Study the drawing (mm; zero at the part's minimum x, y, z) and answer. A direction names the side the tool comes from. Round coordinates to 2 decimals unless told otherwise and drop trailing zeros. Order: outer loops, then holes, each group sorted by start corner. A loop starts at its lowest first (then second) coordinate and runs counter-clockwise, first axis right, second up. Notation, with made-up numbers: M -26.75,71.5 L -12.75,71.5 A8 cw -12.75,83.5 Z; hole C 65.25,49.25 d9. An arc over 180 degrees is marked long. Put each result on its own line as item: value. Start each with the question number.
1. The mould has two halves that part along Y. Classify the marked faces 1, 2 and 3: +Y half, -Y half, draft (parallel to the pull), parting line (faces both ways), or undercut.
2. The part is cut by section A-A (z = 17). Give the vertices of the cut face in (x, y), then the cut area to 3 significant figures.
3. The part is cut by section B-B (x = 5). Give the vertices of the cut face in (y, z), then the cut area to 3 significant figures.
4. Each of these flat-tipped pins is pushed along its axis until it touches: pin 1 Ø5 at (y, z) = (11.5, 15.5) entering from -X; pin 2 Ø3 at (y, z) = (6, 20) entering from +X; pin 3 Ø5 at (x, y) = (24, 8) entering from -Z; pin 4 Ø3 at (x, z) = (6.5, 17.5) entering from +Y. Where does it stop, or does it pass through?
5. The part is cut by section C-C (z = 10.25). Give the vertices of the cut face in (x, y).
6. Which of the six approach directions +Z, -Z, +X, -X, +Y, -Y give full straight-line access (tool end or side, diameter ignored) to the marked faces 4, 5 and 6?
7. Consider line 1 (X direction, y = 1, z = 17); line 2 (X direction, y = 10, z = 17.75); line 3 (X direction, y = 5, z = 11.25). Determine where each line is inside the solid, lowest interval first.
8. The part is cut by section D-D (y = 14). Give the vertices of the cut face in (x, z), then the cut area to 3 significant figures.
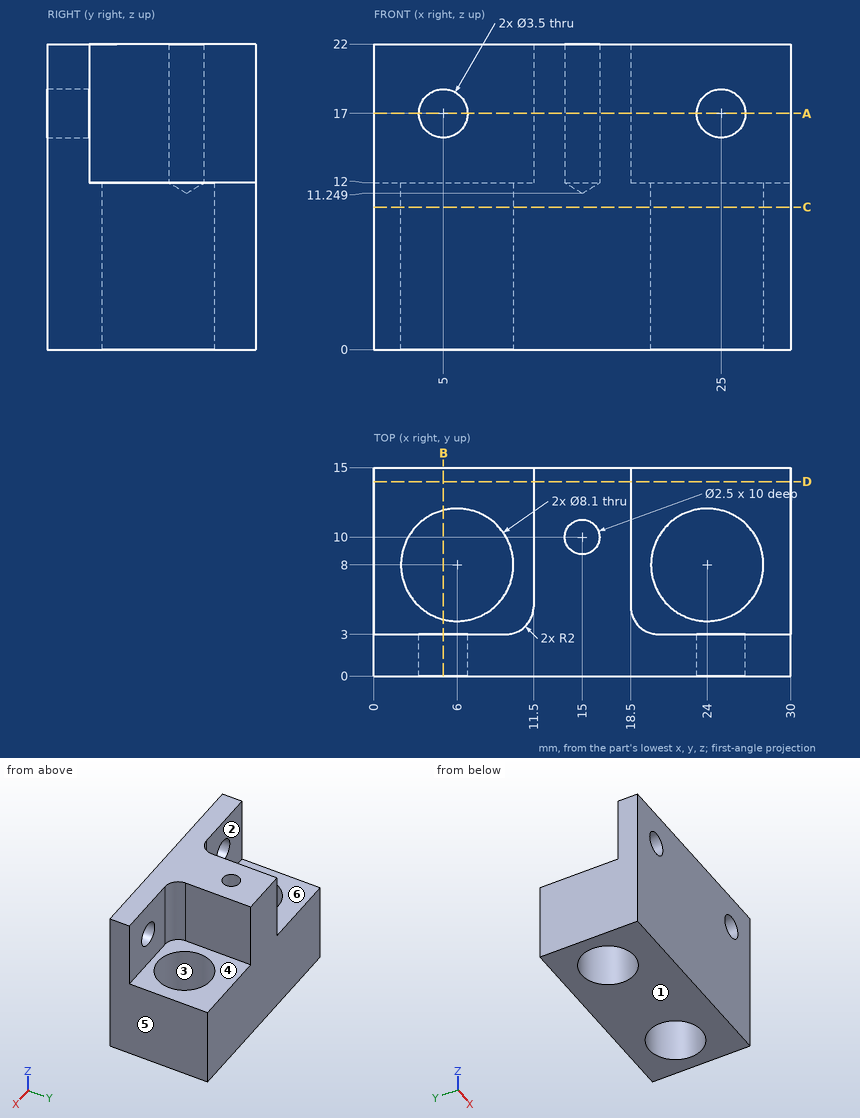
Resolved:
1. face 1: draft
1. face 2: +Y half
1. face 3: undercut
2. outline: M 0,0 L 3.25,0 L 3.25,3 L 0,3 Z; M 6.75,0 L 23.25,0 L 23.25,3 L 20.5,3 A2 cw 18.5,5 L 18.5,15 L 11.5,15 L 11.5,5 A2 cw 9.5,3 L 6.75,3 Z; M 26.75,0 L 30,0 L 30,3 L 26.75,3 Z; hole C 15,10 d2.5
2. area: 150 mm2
3. outline: M 0,0 L 4.08,0 L 4.08,12 L 3,12 L 3,15.25 L 0,15.25 Z; M 0,18.75 L 3,18.75 L 3,22 L 0,22 Z; M 11.92,0 L 15,0 L 15,12 L 11.92,12 Z
3. area: 105 mm2
4. pin 1: x = 11.5
4. pin 2: x = 18.56
4. pin 3: through
4. pin 4: y = 3
5. outline: M 0,0 L 30,0 L 30,15 L 0,15 Z; hole C 6,8 d8.1; hole C 24,8 d8.1
6. face 4: +Z, +X, +Y
6. face 5: +Z, -Z, +X, +Y, -Y
6. face 6: +Z, -X, +Y
7. line 1: 0 to 3.25, 6.75 to 23.25, 26.75 to 30
7. line 2: 11.5 to 13.75, 16.25 to 18.5
7. line 3: 0 to 3.28, 8.72 to 21.28, 26.72 to 30
8. outline: M 0,0 L 30,0 L 30,12 L 18.5,12 L 18.5,22 L 11.5,22 L 11.5,12 L 0,12 Z
8. area: 430 mm2
